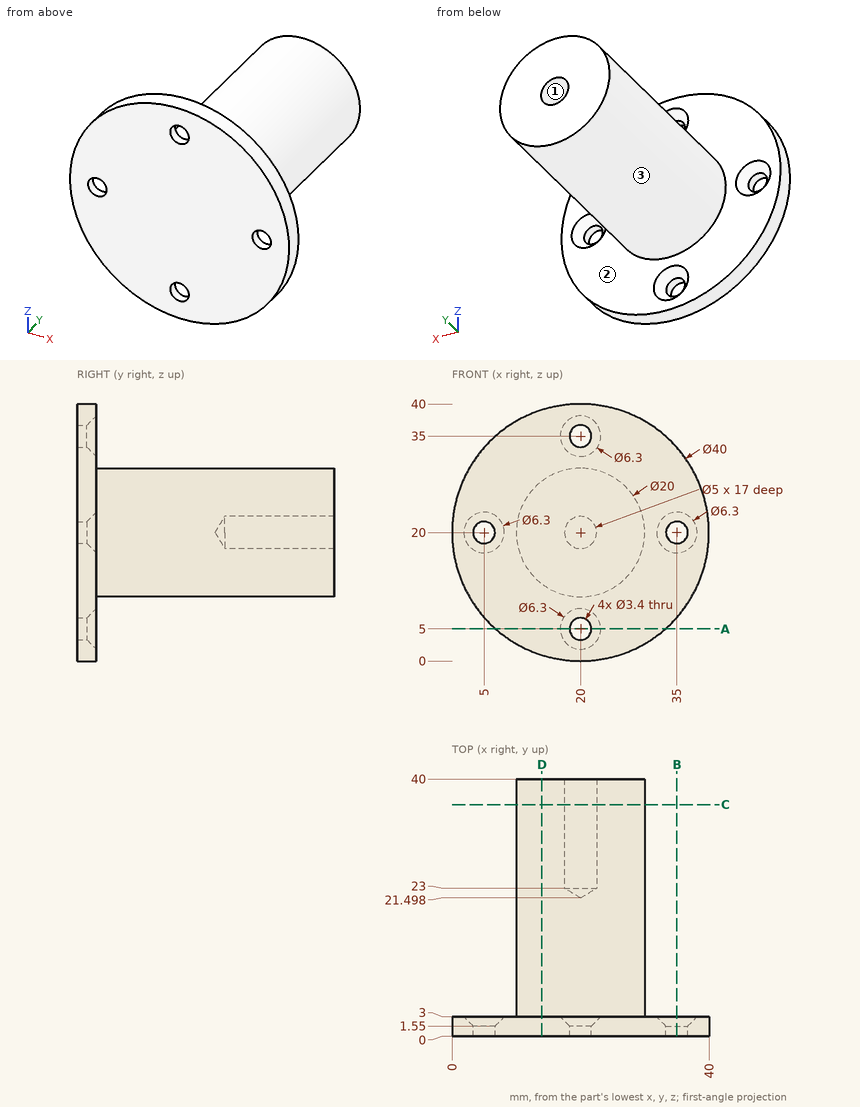
Source: three-view drawing plus pictorial views. Frame: mm from the lowest corner of the part. Coordinates: 2 decimals unless noted, no trailing zeros. Order: outer loops, then holes, each group sorted by start corner. A loop starts at its lowest first (then second) coordinate and runs counter-clockwise, first axis right, second up. Notation, with made-up numbers: M 47.25,64 L 66.25,64 A7 ccw 66.25,76 Z; hole C 23.5,67.25 d4. An arc over 180 degrees is marked long. One line per question, with ' | ' between items.
Item 1: Section B-B (x = 35). Output: boundary loops of the cut face in (y, z).
Geometry results:
outline: M 0,6.77 L 3,6.77 L 3,16.85 L 1.55,18.3 L 0,18.3 Z; M 0,21.7 L 1.55,21.7 L 3,23.15 L 3,33.23 L 0,33.23 Z
Item 2: Ray query, line 1 along Z through (x, y) = (20, 34); line 2 along Y through (x, z) = (28, 11.5). Return the intervals inside material, ascending.
Geometry results:
line 1: z = 10 to 17.5, 22.5 to 30 | line 2: y = 0 to 3
Item 3: Pin query (flat end, axial travel): pin 1 (4 mm diameter, centred on x = 11, y = 32, fed in from +Z); pin 2 (1.5 mm diameter, centred on x = 29.5, y = 12.5, fed in from -Z); pin 3 (4 mm diameter, centred on x = 32, z = 33.5, fed in from +Y). Return the tip coordinate at first contact, or that it passes through.
Geometry results:
pin 1: stops at z = 27.14 | pin 2: stops at z = 15.16 | pin 3: stops at y = 3
Item 4: Section A-A (z = 5). Output: boundary loops of the cut face in (x, y), then the cut area to 3 significant figures.
Geometry results:
outline: M 6.77,0 L 18.3,0 L 18.3,1.55 L 16.85,3 L 6.77,3 Z; M 21.7,0 L 33.23,0 L 33.23,3 L 23.15,3 L 21.7,1.55 Z | area: 67.1 mm^2
Item 5: Section D-D (x = 14). Output: boundary loops of the cut face in (y, z).
Geometry results:
outline: M 0,0.92 L 3,0.92 L 3,12 L 40,12 L 40,28 L 3,28 L 3,39.08 L 0,39.08 Z
Item 6: Draft query along Z for the marked faces 1, 2 and 3. Return one class per face: released by +Z, released by -Z, zero draft, split by the parting line, or undercut.
Geometry results:
face 1: undercut | face 2: zero draft | face 3: split by the parting line
Item 7: Section C-C (y = 36). Output: boundary loops of the cut face in (x, z), then the cut area to 4 significant figures.
Geometry results:
outline: C 20,20 d20; hole C 20,20 d5 | area: 294.5 mm^2
